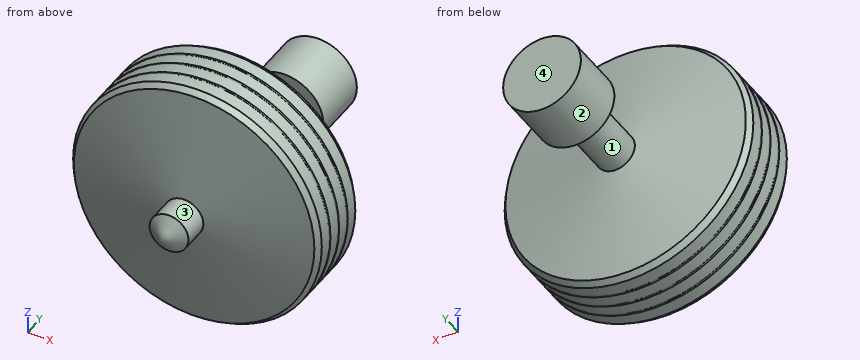
Autodesk Inventor part; units mm, degrees
ref_plane "YZ Plane" through (0, 0, 0) normal (1, 0, 0) x (0, 1, 0)
ref_plane "XZ Plane" through (0, 0, 0) normal (0, 1, 0) x (-1, 0, 0)
ref_plane "XY Plane" through (0, 0, 0) normal (0, 0, 1) x (1, 0, 0)
sketch "Sketch1" plane through (0, 0, 0) normal (0, 0, 1) x (1, 0, 0)
  line L0 (0, 0) -> (0, 28.575)
  line L1 (0, 0) -> (0, -6.35)
  line L2 (0, 28.575) -> (0, 38.1)
  line L3 (6.35, 28.575) -> (6.35, 38.1)
  line L4 (6.35, 38.1) -> (0, 38.1)
  line L5 (3.175, 17.0324) -> (0, 17.0324) construction
  line L6 (6.35, 28.575) -> (3.175, 28.575)
  line L7 (3.175, 28.575) -> (0, 28.575) construction
  line L8 (0, 0) -> (3.175, 0) construction
  line L9 (3.175, 0) -> (17.91, 0) construction
  line L10 (19.6531, 2.9055) -> (20.32, 3.858)
  line L11 (0, -6.35) -> (3.175, -4.2333)
  line L12 (3.175, -4.2333) -> (3.175, 0)
  line L13 (3.175, 0) -> (19.6531, 2.9055)
  line L14 (3.175, 28.575) -> (3.175, 17.2411)
  line L15 (20.32, 13.383) -> (19.6531, 14.3355)
  line L16 (19.6531, 14.3355) -> (3.175, 17.2411)
  line L17 (20.32, 8.7793) -> (20.1613, 8.6205) construction
  line L18 (20.1613, 8.6205) -> (20.32, 8.4618) construction
  arc A0 (6.35, 38.1) -> (0, 40.0262) centre (0, 28.5962) ccw
  line L19 (20.32, 6.3187) -> (20.1612, 6.1599) construction
  line L20 (20.1612, 6.1599) -> (20.32, 6.0012) construction
  line L21 (20.32, 10.9224) -> (20.1612, 11.0812) construction
  line L22 (20.1612, 11.0812) -> (20.32, 11.2399) construction
  line L23 (20.32, 3.858) -> (20.32, 6.0012)
  line L24 (20.32, 6.3187) -> (20.32, 8.4618)
  line L25 (20.32, 8.7793) -> (20.32, 10.9224)
  line L26 (20.32, 11.2399) -> (20.32, 13.383)
  line L27 (20.32, 6.0012) -> (20.32, 6.3187) construction
  line L28 (20.32, 8.4618) -> (20.32, 8.7793) construction
  line L29 (20.32, 10.9224) -> (20.32, 11.2399) construction
  arc A1 (20.32, 11.2399) -> (20.32, 10.9224) centre (20.4787, 11.0812) ccw
  arc A2 (20.32, 8.7793) -> (20.32, 8.4618) centre (20.4787, 8.6205) ccw
  arc A3 (20.32, 6.3187) -> (20.32, 6.0012) centre (20.4787, 6.1599) ccw
  dimension "d5" = 44.45
  dimension "d6" = 9.525
  dimension "d7" = 6.35
  dimension "d12" = 2.1167
  dimension "d13" = 3.175
  dimension "d15" = 4.2333
  dimension "d24" = 10
  dimension "d28" = 3.175
  dimension "d31" = 110
  dimension "d32" = 100
  dimension "d35" = 11.43
  dimension "d36" = 0.3175
  dimension "d37" = 9.525
  dimension "d40" = 11.43
  dimension "d42" = 20.32
revolve "Revolution1" add sketch "Sketch1" angle 360 about axis through (0, 28.575, 0) along (0, -1, 0)
properties part number "Top1"
Source: CAD feature listing. Evaluate the final solid. Frame: model axes, mm. Face numbers are marked on the shaded views. A direction names the side the tool comes from. Round coordinates to 2 decimals unless told otherwise and drop trailing zeros. Answer as a JSON object with one key per item and string values. Group by question number.
Q1. Access query for the marked faces 1, 2, 3 and 4. Directions: +Z, -Z, +X, -X, +Y, -Y. A direction counts if a zero-diameter tool reaches every point of the face in a straight line with its end or side. Return the directions, or none.
Q2. Contact query for flat-ended pins moving along their axis: P1, Ø10, axis at x = 1, z = 14.5, coming from the -Y side; P2, Ø2, axis at x = 0.5, y = 28, coming from the +Z side; P3, Ø6, axis at x = -14, z = 0.5, coming from the -Y side. Output: stop coordinate, or through.
Q3. Ray query, line 1 (Z direction, x = 2.5, y = 17.5); line 2 (X direction, y = 3, z = -3.5); line 3 (Z direction, x = -12, y = 3). Return the intervals inside material, ascending. Write a range as from..to.
Completed:
{
 "1": {"face 1": "none", "face 2": "+Y", "face 3": "-Y", "face 4": "+Z, -Z, +X, -X, +Y"},
 "2": {"P1": "y = 1.12", "P2": "z = 6.35", "P3": "y = 1.38"},
 "3": {"line 1": "-1.96..1.96", "line 2": "-19.41..19.41", "line 3": "-15.65..15.65"}
}
